Verification items for the finished model (mm, model axes). A direction names the side the tool comes from. Give positions to 0.01 mm unless a question says otherwise; leave off trailing zeros. Loops run counter-clockwise (first coordinate to the right, second up) from the corner with the lowest first, then second, coordinate; pieces in that order, holes last. Notation, with made-up numbers: (83.25, 55) -> (131.25, 55) arc R23 cw to (131.25, 92) -> close; hole circle Ø4 at (75.5, -9). An arc over 180 degrees is marked (long way). Answer in a Markdown table with one row per item. Add a question column.
Q1. Section check A-A on z = 0. Enter the section's corners in (x, y).
Q2. Section check B-B on x = 0. Enter the section's corners in (y, z).
Q3. Material ranges on probe 1 along Z at (x, y) = (0, 55); probe 2 along X at (y, z) = (93.5, -29), recorded low to high.
Q4. Gauge pin test, flat ends, axial feed: P1, Ø1, axis at y = 112.5, z = -12.5, coming from the +X side; P2, Ø6, axis at x = 17.5, y = 31.5, coming from the -Z side; P3, Ø6, axis at x = -8, y = 33, coming from the -Z side. Record the tip position at first contact, or that the pin passes through.
Q5. Set-up check for faces 1 (the face through (37.29, 35.58, 0.23)), 2 (the face through (35.23, 72.87, 14.61)): record each of +Z, -Z, +X, -X, +Y, -Y from which the full face is reachable in a straight line by a thin tool's end or side.
Q6. Section check D-D on y = 118. Enter the section's corners in (x, z) (1 decimal).
Q7. Section check C-C on z = 15. Enter the section's corners in (x, y), and give its area (3 significant figures).
Q8. Release check for a two-part mould opening along Y. For faces 3 (the face through (-18.847, 35.578, 32.179)), 4 (the face through (31, 147.815, 20)), 5 (the face through (31, 0, 20)) record: pulls with the +Y half, pulls with the -Y half, needs draft (parallel to the pull), parting line crosses it, or undercut.
```python
from build123d import *

# Parameters (mm, degrees)
SKETCH1_R           = 38.1381
SKETCH1_R_2         = 36.5125
BOSS_EXTRUDE1_DEPTH = 147.8153
CUT_EXTRUDE1_START  = -1.669304
SKETCH2_R           = 1.7859375
CUT_EXTRUDE1_DEPTH  = 1.669304
CIRPATTERN1_COUNT   = 3


with BuildPart() as part:
    # Sketch1 → Boss-Extrude1 (new body)
    with BuildSketch(Plane(origin=(0, 0, 0), x_dir=(1, 0, 0), z_dir=(0, 1, 0))):
        Circle(SKETCH1_R)
        Circle(SKETCH1_R_2, mode=Mode.SUBTRACT)
    extrude(amount=BOSS_EXTRUDE1_DEPTH)

    # Sketch2 → Cut-Extrude1 (cut)
    with BuildSketch(Plane(origin=(38.1381, 0, 0), x_dir=(0, 0, -1), z_dir=(1, 0, 0)).offset(CUT_EXTRUDE1_START)):
        with Locations((0, 33.8074)):
            Circle(SKETCH2_R)
    cut_extrude1 = extrude(amount=CUT_EXTRUDE1_DEPTH, mode=Mode.SUBTRACT)

    # CirPattern1: Cut-Extrude1 ×3 about axis
    cirpattern1_axis = Axis((0, 155.08605, 0), (0, -1, 0))
    for i in range(1, CIRPATTERN1_COUNT):
        add(cut_extrude1.rotate(cirpattern1_axis, i * 360 / CIRPATTERN1_COUNT), mode=Mode.SUBTRACT)


solid = part.part
```
Taken from the geometry:
| question | item | result |
|---|---|---|
| 1 | outline | (-38.14, 0) -> (-36.51, 0) -> (-36.51, 147.82) -> (-38.14, 147.82) -> close; (36.51, 0) -> (38.14, 0) -> (38.14, 32.02) -> (36.51, 32.02) -> close; (36.51, 35.59) -> (38.14, 35.59) -> (38.14, 147.82) -> (36.51, 147.82) -> close |
| 2 | outline | (0, -38.14) -> (147.82, -38.14) -> (147.82, -36.51) -> (0, -36.51) -> close; (0, 36.51) -> (147.82, 36.51) -> (147.82, 38.14) -> (0, 38.14) -> close |
| 3 | probe 1 | z = -38.14 to -36.51, 36.51 to 38.14 |
| 3 | probe 2 | x = -24.77 to -22.18, 22.18 to 24.77 |
| 4 | P1 | stops at x = 36.2 |
| 4 | P2 | stops at z = -35.27 |
| 4 | P3 | stops at z = -37.81 |
| 5 | face 1 | +X |
| 5 | face 2 | +Y, -Y |
| 6 | outline | circle Ø76.3 at (0, 0); hole circle Ø73 at (0, 0) |
| 7 | outline | (-35.06, 0) -> (-33.29, 0) -> (-33.29, 147.82) -> (-35.06, 147.82) -> close; (33.29, 0) -> (35.06, 0) -> (35.06, 147.82) -> (33.29, 147.82) -> close |
| 7 | area | 525 mm² |
| 8 | face 3 | undercut |
| 8 | face 4 | pulls with the +Y half |
| 8 | face 5 | pulls with the -Y half |
